Design review of the part shown in the three views and the two pictorial views. Dimensions are in mm from the part's minimum x, y and z. Round coordinates to 2 decimals unless told otherwise and drop trailing zeros. Write each loop counter-clockwise with the first axis right and the second up, starting at its lowest first coordinate (ties: lowest second). Pieces come first, ordered by that corner, then holes. Notation, with made-up numbers: (84, 46.5) -> (94, 46.5) arc R30 cw to (94, 78.5) -> close; hole circle Ø7 at (87.25, 84.25). An arc over 180 degrees is marked (long way). Return JSON: item names as keys, results as strings. Group by question number.
1. Mouldability with a two-part tool opening along X and no side actions: class the marked faces 1, 2 and 3 as pulls with the +X half, pulls with the -X half, needs draft (parallel to the pull), parting line crosses it, or undercut.
2. Take a section at C-C, the plane x = 9. Write out the cut boundary in (y, z), then the cut area to 3 significant figures.
3. Take a section at A-A, the plane x = 5. Write out the cut boundary in (y, z).
4. Clearance check with a flat-ended pin moving along its axis: P1, Ø2, axis at y = 5, z = 5, coming from the -X side. State where the tip first meets the part, or that it passes through.
5. For line 1 along Z through (x, y) = (8.1, 5), list the stretches that pass through material, from the lowest coordinate up. Write a range as from..to.
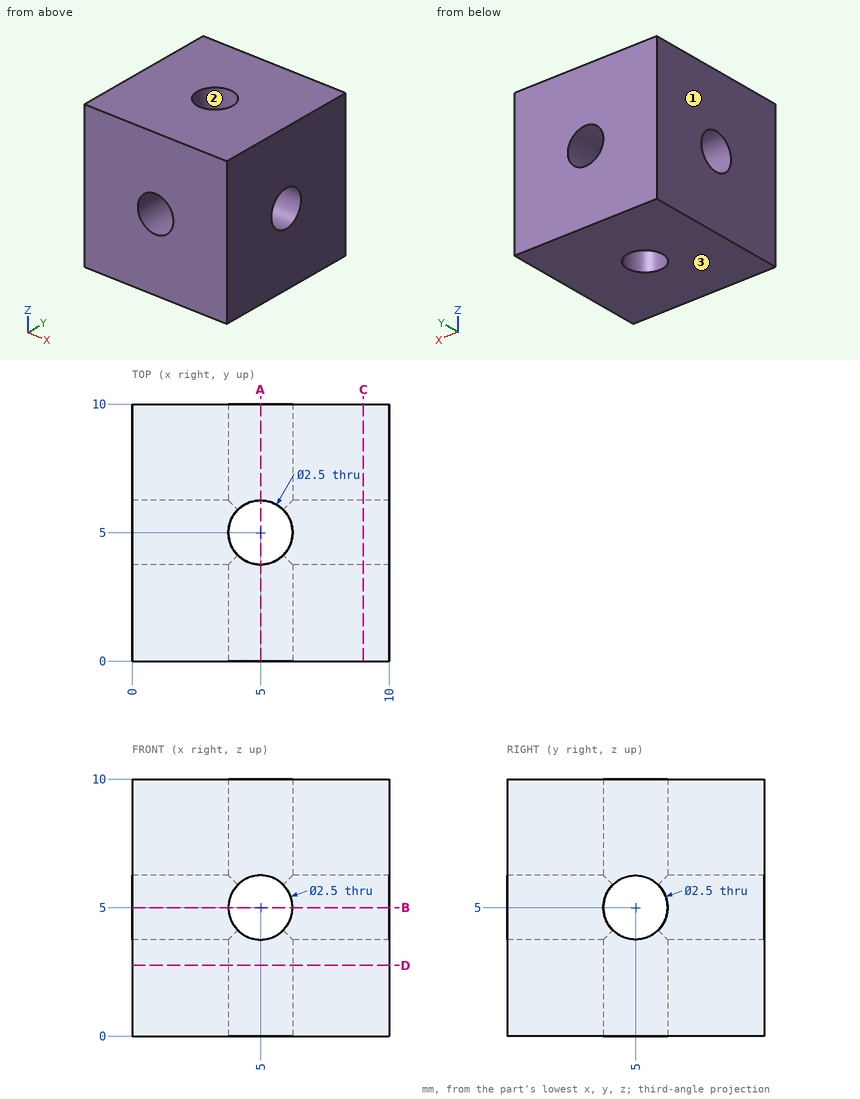
Output:
{
 "1": {"face 1": "pulls with the -X half", "face 2": "undercut", "face 3": "needs draft"},
 "2": {"outline": "(0, 0) -> (10, 0) -> (10, 10) -> (0, 10) -> close; hole circle Ø2.5 at (5, 5)", "area": "95.1 mm^2"},
 "3": {"outline": "(0, 0) -> (3.75, 0) -> (3.75, 3.75) -> (0, 3.75) -> close; (0, 6.25) -> (3.75, 6.25) -> (3.75, 10) -> (0, 10) -> close; (6.25, 0) -> (10, 0) -> (10, 3.75) -> (6.25, 3.75) -> close; (6.25, 6.25) -> (10, 6.25) -> (10, 10) -> (6.25, 10) -> close"},
 "4": {"P1": "passes through"},
 "5": {"line 1": "z = 0..3.75, 6.25..10"}
}
